Here's how the part is built. I have some questions about the finished solid (model axes, mm). A direction names the side the tool comes from. Round coordinates to 2 decimals unless told otherwise and drop trailing zeros. Write each loop counter-clockwise with the first axis right and the second up, starting at its lowest first coordinate (ties: lowest second). Pieces come first, ordered by that corner, then holes. Notation, with made-up numbers: (12.25, 29.25) -> (38.25, 29.25) arc R33 cw to (38.25, 58.25) -> close; hole circle Ø6 at (45.5, -24). An arc over 180 degrees is marked (long way). Answer in a Markdown table with one row per item.
from build123d import *

# Parameters (mm, degrees)
SKETCH1_W           = 115.2652
SKETCH1_H           = 114.935
SKETCH1_W_2         = 3.175
BOSS_EXTRUDE1_DEPTH = 3.175
SKETCH1_3_W         = 3.175
SKETCH1_3_H         = 114.935
BOSS_EXTRUDE2_DEPTH = 12.7
FILLET1_R           = 8.10006
CHAMFER1_SIZE       = 1.5
FILLET2_R           = 1


with BuildPart() as part:
    # Sketch1 → Boss-Extrude1 (new body)
    with BuildSketch(Plane(origin=(0, 0, 0), x_dir=(1, 0, 0), z_dir=(0, 1, 0))):
        Rectangle(SKETCH1_W, SKETCH1_H)
        with BuildLine():
            ThreePointArc((-35.2425, 51.1175), (-37.48756403, 50.18756403), (-38.4175, 47.9425))
            Line((-38.4175, 47.9425), (-38.4175, -47.9425))
            ThreePointArc((-38.4175, -47.9425), (-37.48756403, -50.18756403), (-35.2425, -51.1175))
            Line((-35.2425, -51.1175), (35.2425, -51.1175))
            ThreePointArc((35.2425, -51.1175), (37.48756403, -50.18756403), (38.4175, -47.9425))
            Line((38.4175, -47.9425), (38.4175, 47.9425))
            ThreePointArc((38.4175, 47.9425), (37.48756403, 50.18756403), (35.2425, 51.1175))
            Line((35.2425, 51.1175), (-35.2425, 51.1175))
        make_face(mode=Mode.SUBTRACT)
        with Locations((-59.2201, 0)):
            Rectangle(SKETCH1_W_2, SKETCH1_H)
        with Locations((59.2201, 0)):
            Rectangle(SKETCH1_W_2, SKETCH1_H)
    extrude(amount=BOSS_EXTRUDE1_DEPTH)

    # Sketch1_3 → Boss-Extrude2 (add)
    with BuildSketch(Plane(origin=(0, 0, 0), x_dir=(1, 0, 0), z_dir=(0, 1, 0))):
        with Locations((59.2201, 0)):
            Rectangle(SKETCH1_3_W, SKETCH1_3_H)
        with Locations((-59.2201, 0)):
            Rectangle(SKETCH1_3_W, SKETCH1_3_H)
    extrude(amount=-BOSS_EXTRUDE2_DEPTH)

    # Fillet1
    fillet1_edges = [part.edges().sort_by_distance(p)[0] for p in [
        (57.6326, 0, 0),
        (-57.6326, 0, 0),
    ]]
    fillet(fillet1_edges, radius=FILLET1_R)

    # Chamfer1
    chamfer1_edges = [part.edges().sort_by_distance(p)[0] for p in [
        (57.6326, -12.7, 0),
        (57.6326, -10.40003, 57.4675),
        (57.6326, -10.40003, -57.4675),
        (-57.6326, -10.40003, -57.4675),
        (-57.6326, -10.40003, 57.4675),
        (-57.6326, -12.7, 0),
        (0, 0, -57.4675),
        (0, 0, 57.4675),
        (-55.260147354, -2.372452646, 57.4675),
        (-55.260147354, -2.372452646, -57.4675),
        (55.260147354, -2.372452646, 57.4675),
        (55.260147354, -2.372452646, -57.4675),
    ]]
    chamfer(chamfer1_edges, length=CHAMFER1_SIZE)

    # Fillet2
    fillet2_edges = [part.edges().sort_by_distance(p)[0] for p in [
        (-60.8076, -4.7625, 57.4675),
        (-60.8076, -4.7625, -57.4675),
        (60.8076, -4.7625, 57.4675),
        (60.8076, -4.7625, -57.4675),
    ]]
    fillet(fillet2_edges, radius=FILLET2_R)


solid = part.part
1) I need wall thicknesses on line 1 (X direction, y = -9, z = -23); line 2 (X direction, y = 1.75, z = 48); line 3 (Y direction, x = 47.5, z = 0.5) (3 decimals). Which ranges of each line are inside material? Lowest first, please. Write a range as [from, to].
Response:
| item | result |
|---|---|
| line 1 | x = [-60.81, -57.63], [57.63, 60.81] |
| line 2 | x = [-60.81, -38.42], [38.42, 60.81] |
| line 3 | y = [0, 3.175] |
2) Which directions (+Z, -Z, +X, -X, +Y, -Y) give clear straight access to the entire face, cutting with the end or side of a thin tool? Please do faces 1 (the face through (-57.633, -10, 1)), 2 (the face through (55.38, -2.12, -56.23)), 3 (the face through (-55.51, -2.25, 56.23)), 4 (the face through (0, 2, -51.118)).
Response:
| item | result |
|---|---|
| face 1 | +Z, -Z, -Y |
| face 2 | -Z, -Y |
| face 3 | +Z, -Y |
| face 4 | +Y, -Y |
3) I want a section at B-B, the plane x = -13.5. List the corners of the cut face in (y, z) for me (1 decimal), and give its area (3 significant figures).
Response:
| item | result |
|---|---|
| outline | (0, -56) -> (1.5, -57.5) -> (3.2, -57.5) -> (3.2, -51.1) -> (0, -51.1) -> close; (0, 51.1) -> (3.2, 51.1) -> (3.2, 57.5) -> (1.5, 57.5) -> (0, 56) -> close |
| area | 38.1 mm^2 |
4) For pin 1 (1 mm diameter, centred on x = -39.5, z = -13, fed in from -Y), with a flat end and sliding along its axis, tell me the tip position at first contact or that it passes through.
Response:
| item | result |
|---|---|
| pin 1 | stops at y = 0 |
5) I want a section at A-A, the plane z = -27. List the corners of the cut face in (x, y) for me (1 decimal).
Response:
| item | result |
|---|---|
| outline | (-60.8, -12.7) -> (-59.1, -12.7) -> (-57.6, -11.2) -> (-57.6, -8.1) arc R8.1 cw to (-49.5, 0) -> (-38.4, 0) -> (-38.4, 3.2) -> (-60.8, 3.2) -> close; (38.4, 0) -> (49.5, 0) arc R8.1 cw to (57.6, -8.1) -> (57.6, -11.2) -> (59.1, -12.7) -> (60.8, -12.7) -> (60.8, 3.2) -> (38.4, 3.2) -> close |
6) We'd pull the mould along X, two halves only. Please class faces 5 (the face through (60.808, -5, 1)), 6 (the face through (-60.808, -5, 1)), 7 (the face through (37.512, 1.565, -50.163)), 8 (the face through (-41, 3.175, -1)): +X half, -X half, draft (parallel to the pull), parting line (faces both ways), or undercut.
Response:
| item | result |
|---|---|
| face 5 | +X half |
| face 6 | -X half |
| face 7 | undercut |
| face 8 | draft |
7) I want a section at C-C, the plane x = -42.5. List the corners of the cut face in (y, z) for me (1 decimal).
Response:
| item | result |
|---|---|
| outline | (0, -56) -> (1.5, -57.5) -> (3.2, -57.5) -> (3.2, 57.5) -> (1.5, 57.5) -> (0, 56) -> close |
